The model under review builds one solid part; all positions refer to its coordinate system, in mm. A direction names the side the tool comes from. Round coordinates to 2 decimals unless told otherwise and drop trailing zeros. Write each loop counter-clockwise with the first axis right and the second up, starting at its lowest first coordinate (ties: lowest second). Pieces come first, ordered by that corner, then holes. Notation, with made-up numbers: (-33.75, -6.5) -> (-17.75, -6.5) arc R15 ccw to (-17.75, 4.5) -> close; hole circle Ø4 at (47, 48). An arc over 180 degrees is marked (long way). Use CSV: the item, a comma, the result in double quotes. Start each with the question number.
1) Wall thickness on probe 1 along X at (y, z) = (-34, -1.5); probe 2 along X at (y, z) = (29, 96.5); probe 3 along Y at (x, z) = (-20.5, 54.5): over which ranges is each line inside the solid? List them lowest first. Write a range as [from, to].
2) Take a section at A-A, the plane y = 8. Give the boundary of the cut face in (x, z), then the cut area to 3 significant figures.
3) Machinability: for faces 3 (the face through (24.25, 38, 1)), 4 (the face through (15.75, -38, 1)), 5 (the face through (-38, -15.75, 1)), 6 (the face through (38, -15.75, 1)), 7 (the face through (16.15, 16.07, 1.49)), which of the approach directions +Z, -Z, +X, -X, +Y, -Y give a long, thin tool a straight path to every point of the face, cutting with its end or side? Answer none if there is none.
4) Mouldability with a two-part tool opening along Y and no side actions: class faces 1 (the face through (-12.85, 32, 1)), 2 (the face through (-15, -21, -106.5)) as released by +Y, released by -Y, zero draft, split by the parting line, or undercut.
5) Take a section at B-B, the plane z = -80.5. State how many separate pieces and enclosed holes the cut face has, then the cut area to 3 significant figures.
6) For pin 1 Ø2 at (y, z) = (-21, 22.5) entering from +X; pin 2 Ø5.5 at (x, z) = (23.5, -44) entering from +Y; pin 3 Ø1.5 at (x, z) = (22, -76.5) entering from -Y, all flat-tipped, find the tip position at first contact; note any pin that passes through.
from build123d import *

# Parameters (mm, degrees)
SKETCH_1_R      = 3.4
SKETCH_1_R_2    = 4
EXTRUDE_1_DEPTH = 106.5


with BuildPart() as part:
    # 草图1 → 凸台-拉伸1 (new, symmetric)
    with BuildSketch(Plane.XY):
        with BuildLine():
            Line((-40, 40), (-24.25, 40))
            Line((-24.25, 40), (-24.25, 36))
            Line((-24.25, 36), (-27.15, 36))
            Line((-27.15, 36), (-27.15, 29))
            ThreePointArc((-27.15, 29), (-20, 25.5), (-12.85, 29))
            Line((-12.85, 29), (-12.85, 36))
            Line((-12.85, 36), (-15.75, 36))
            Line((-15.75, 36), (-15.75, 40))
            Line((-15.75, 40), (15.75, 40))
            Line((15.75, 40), (15.75, 36))
            Line((15.75, 36), (12.85, 36))
            Line((12.85, 36), (12.85, 29))
            ThreePointArc((12.85, 29), (20, 25.5), (27.15, 29))
            Line((27.15, 29), (27.15, 36))
            Line((27.15, 36), (24.25, 36))
            Line((24.25, 36), (24.25, 40))
            Line((24.25, 40), (40, 40))
            Line((40, 40), (40, 24.25))
            Line((40, 24.25), (36, 24.25))
            Line((36, 24.25), (36, 27.15))
            Line((36, 27.15), (29, 27.15))
            ThreePointArc((29, 27.15), (25.5, 20), (29, 12.85))
            Line((29, 12.85), (36, 12.85))
            Line((36, 12.85), (36, 15.75))
            Line((36, 15.75), (40.000271684, 15.75))
            Line((40.000271684, 15.75), (40.000271684, -15.75))
            Line((40.000271684, -15.75), (36, -15.75))
            Line((36, -15.75), (36, -12.85))
            Line((36, -12.85), (29, -12.85))
            ThreePointArc((29, -12.85), (25.5, -20), (29, -27.15))
            Line((29, -27.15), (36, -27.15))
            Line((36, -27.15), (36, -24.25))
            Line((36, -24.25), (40, -24.25))
            Line((40, -24.25), (40, -40))
            Line((40, -40), (24.25, -40))
            Line((24.25, -40), (24.25, -36))
            Line((24.25, -36), (27.15, -36))
            Line((27.15, -36), (27.15, -29))
            ThreePointArc((27.15, -29), (20, -25.5), (12.85, -29))
            Line((12.85, -29), (12.85, -36))
            Line((12.85, -36), (15.75, -36))
            Line((15.75, -36), (15.75, -40))
            Line((15.75, -40), (-15.75, -40))
            Line((-15.75, -40), (-15.75, -36))
            Line((-15.75, -36), (-12.85, -36))
            Line((-12.85, -36), (-12.85, -29))
            ThreePointArc((-12.85, -29), (-20, -25.5), (-27.15, -29))
            Line((-27.15, -29), (-27.15, -36))
            Line((-27.15, -36), (-24.25, -36))
            Line((-24.25, -36), (-24.25, -40))
            Line((-24.25, -40), (-40, -40))
            Line((-40, -40), (-40, -24.25))
            Line((-40, -24.25), (-36, -24.25))
            Line((-36, -24.25), (-36, -27.15))
            Line((-36, -27.15), (-29, -27.15))
            ThreePointArc((-29, -27.15), (-25.5, -20), (-29, -12.85))
            Line((-29, -12.85), (-36, -12.85))
            Line((-36, -12.85), (-36, -15.75))
            Line((-36, -15.75), (-40.000271684, -15.75))
            Line((-40.000271684, -15.75), (-40.000271684, 15.75))
            Line((-40.000271684, 15.75), (-36, 15.75))
            Line((-36, 15.75), (-36, 12.85))
            Line((-36, 12.85), (-29, 12.85))
            ThreePointArc((-29, 12.85), (-25.5, 20), (-29, 27.15))
            Line((-29, 27.15), (-36, 27.15))
            Line((-36, 27.15), (-36, 24.25))
            Line((-36, 24.25), (-40, 24.25))
            Line((-40, 24.25), (-40, 40))
        make_face()
        with Locations((-20, 20)):
            Circle(SKETCH_1_R, mode=Mode.SUBTRACT)
        with Locations((-33.575, 33.575)):
            Circle(SKETCH_1_R_2, mode=Mode.SUBTRACT)
        with Locations((33.575, 33.575)):
            Circle(SKETCH_1_R_2, mode=Mode.SUBTRACT)
        with Locations((20, 20)):
            Circle(SKETCH_1_R, mode=Mode.SUBTRACT)
        with Locations((20, -20)):
            Circle(SKETCH_1_R, mode=Mode.SUBTRACT)
        with Locations((33.575, -33.575)):
            Circle(SKETCH_1_R_2, mode=Mode.SUBTRACT)
        with Locations((-33.575, -33.575)):
            Circle(SKETCH_1_R_2, mode=Mode.SUBTRACT)
        with Locations((-20, -20)):
            Circle(SKETCH_1_R, mode=Mode.SUBTRACT)
        with BuildLine():
            Line((10.35, 37), (-10.35, 37))
            Line((-10.35, 37), (-10.35, 29))
            Line((-10.35, 29), (-14.5, 24.85))
            Line((-14.5, 24.85), (-14.5, 20))
            ThreePointArc((-14.5, 20), (-16.110912703, 16.110912703), (-20, 14.5))
            Line((-20, 14.5), (-24.85, 14.5))
            Line((-24.85, 14.5), (-29, 10.35))
            Line((-29, 10.35), (-37, 10.35))
            Line((-37, 10.35), (-37, -10.35))
            Line((-37, -10.35), (-29, -10.35))
            Line((-29, -10.35), (-24.85, -14.5))
            Line((-24.85, -14.5), (-20, -14.5))
            ThreePointArc((-20, -14.5), (-16.110912703, -16.110912703), (-14.5, -20))
            Line((-14.5, -20), (-14.5, -24.85))
            Line((-14.5, -24.85), (-10.35, -29))
            Line((-10.35, -29), (-10.35, -37))
            Line((-10.35, -37), (10.35, -37))
            Line((10.35, -37), (10.35, -29))
            Line((10.35, -29), (14.5, -24.85))
            Line((14.5, -24.85), (14.5, -20))
            ThreePointArc((14.5, -20), (16.110912703, -16.110912703), (20, -14.5))
            Line((20, -14.5), (24.85, -14.5))
            Line((24.85, -14.5), (29, -10.35))
            Line((29, -10.35), (37, -10.35))
            Line((37, -10.35), (37, 10.35))
            Line((37, 10.35), (29, 10.35))
            Line((29, 10.35), (24.85, 14.5))
            Line((24.85, 14.5), (20, 14.5))
            ThreePointArc((20, 14.5), (16.110912703, 16.110912703), (14.5, 20))
            Line((14.5, 20), (14.5, 24.85))
            Line((14.5, 24.85), (10.35, 29))
            Line((10.35, 29), (10.35, 37))
        make_face(mode=Mode.SUBTRACT)
    extrude(amount=EXTRUDE_1_DEPTH, both=True)


solid = part.part
Values found:
1,probe 1,"[-40, -37.55], [-29.6, -27.15], [-12.85, -10.35], [10.35, 12.85], [27.15, 29.6], [37.55, 40]"
1,probe 2,"[-40, -27.15], [-12.85, -10.35], [10.35, 12.85], [27.15, 40]"
1,probe 3,"[-25.51, -23.36], [-16.64, -14.5], [14.5, 16.64], [23.36, 25.51]"
2,outline,"(-40, -106.5) -> (-37, -106.5) -> (-37, 106.5) -> (-40, 106.5) -> close; (37, -106.5) -> (40, -106.5) -> (40, 106.5) -> (37, 106.5) -> close"
2,area,"1,280 mm²"
3,face 3,"+Z, -Z, +Y"
3,face 4,"+Z, -Z, -Y"
3,face 5,"+Z, -Z, -X"
3,face 6,"+Z, -Z, +X"
3,face 7,"+Z, -Z"
4,face 1,"undercut"
4,face 2,"zero draft"
5,separate pieces,"1"
5,enclosed holes,"9"
5,area,"1,560 mm²"
6,pin 1,"x = 25.72"
6,pin 2,"y = 40"
6,pin 3,"y = -25.93"
